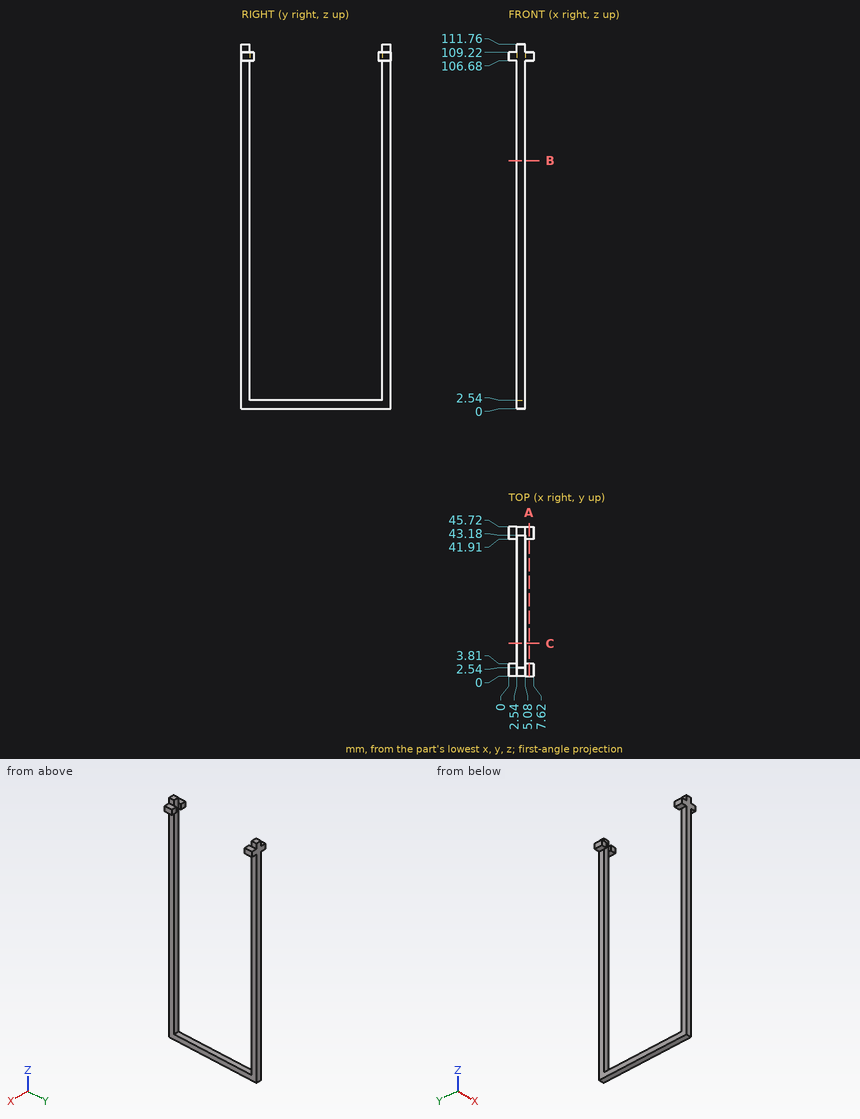
The drawing under review shows one solid part. Ordinate dimensions are in mm from its lowest x, y, z. Coordinates: 2 decimals unless noted, no trailing zeros. Write each loop counter-clockwise with the first axis right and the second up, starting at its lowest first coordinate (ties: lowest second). Pieces come first, ordered by that corner, then holes.
1) Add section B-B (z = 76). Write out the cut boundary in (x, y), plus the area to 3 significant figures.
2) Add section A-A (x = 6.25). Write out the cut boundary in (y, z).
3) Add section C-C (y = 10). Write out the cut boundary in (x, z).
4) To check wall thickness, follow L1, parallel to Y at x = 3.5, z = 37.5; L2, parallel to Z at x = 3.5, y = 43. State the ranges of each line that lie inside material, in increasing order.
5) Insertion check: pin 1 (3 mm diameter, centred on x = 7, y = 44.5, fed in from +Z); pin 2 (2 mm diameter, centred on y = 44.5, z = 110, fed in from +X); pin 3 (12 mm diameter, centred on y = 41, z = 57.5, fed in from -X); pin 4 (0.8 mm diameter, centred on x = 4, y = 21, fed in from +Z). Each pin has a flat end and moves straight along its axis. Give the tip position at first contact, or say it passes through.
Check result:
1. outline: (2.54, 0) - (5.08, 0) - (5.08, 2.54) - (2.54, 2.54) - close; (2.54, 43.18) - (5.08, 43.18) - (5.08, 45.72) - (2.54, 45.72) - close
1. area: 12.9 mm2
2. outline: (0, 106.68) - (3.81, 106.68) - (3.81, 109.22) - (0, 109.22) - close; (41.91, 106.68) - (45.72, 106.68) - (45.72, 109.22) - (41.91, 109.22) - close
3. outline: (2.54, 0) - (5.08, 0) - (5.08, 2.54) - (2.54, 2.54) - close
4. L1: y = 0 to 2.54, 43.18 to 45.72
4. L2: z = 0 to 2.54
5. pin 1: stops at z = 109.22
5. pin 2: stops at x = 7.62
5. pin 3: stops at x = 2.54
5. pin 4: stops at z = 2.54
